Autodesk Inventor part; units mm, degrees
ref_plane "YZ Plane" through (0, 0, 0) normal (1, 0, 0) x (0, 1, 0)
ref_plane "XZ Plane" through (0, 0, 0) normal (0, 1, 0) x (-1, 0, 0)
ref_plane "XY Plane" through (0, 0, 0) normal (0, 0, 1) x (1, 0, 0)
sketch "Sketch1" plane through (0, 0, 0) normal (0, 1, 0) x (-1, 0, 0)
  line L0 (0, 0) -> (89, 0)
  line L1 (89, 0) -> (89, -94)
  line L2 (89, -94) -> (0, -94)
  line L3 (0, -94) -> (0, 0)
  dimension "d0" = 89
  dimension "d1" = 94
extrude "Extrusion1" add sketch "Sketch1" along normal blind 83
sketch "Sketch2" plane through (0, 83, 0) normal (0, 1, 0) x (1, 0, 0)
  line L0 (0, 0) -> (0, 2) construction
  line L1 (0, 0) -> (0, 94)
  line L2 (0, 2) -> (-2, 2) construction
  line L3 (-2, 2) -> (-87, 2)
  line L4 (-87, 2) -> (-87, 92)
  line L5 (-87, 92) -> (-2, 92)
  line L6 (-2, 92) -> (-2, 2)
  dimension "d4" = 2
  dimension "d5" = 2
  dimension "d6" = 85
  dimension "d7" = 90
extrude "Extrusion2" cut sketch "Sketch2" against normal blind 81
sketch "Sketch3" plane through (0, 2, 0) normal (0, 1, 0) x (1, 0, 0)
  line L0 (-87, 2) -> (-87, 92)
  line L1 (-87, 2) -> (-76, 2)
  line L2 (-2, 2) -> (-87, 2)
  line L3 (-76, 2) -> (-17, 2)
  line L4 (-87, 92) -> (-2, 92)
  line L5 (-76, 2) -> (-87, 2)
  line L6 (-87, 2) -> (-87, 92)
  line L7 (-87, 92) -> (-76, 92)
  line L8 (-2, 92) -> (-2, 2)
  line L9 (-17, 2) -> (-2, 2)
  line L10 (-2, 2) -> (-2, 92)
  line L11 (-2, 92) -> (-17, 92)
  line L12 (-87, 2) -> (-87, 17.5)
  line L13 (-87, 17.5) -> (-87, 76.5)
  line L14 (-87, 17.5) -> (-2, 17.5)
  line L15 (-2, 17.5) -> (-2, 2)
  line L16 (-2, 2) -> (-87, 2)
  line L17 (-87, 2) -> (-87, 17.5)
  line L18 (-87, 76.5) -> (-2, 76.5)
  line L19 (-2, 76.5) -> (-2, 92)
  line L20 (-2, 92) -> (-87, 92)
  line L21 (-87, 92) -> (-87, 76.5)
  point P0 (0, 0)
  point P1 (-2, 76.5)
  point P2 (-2, 17.5)
  dimension "d26" = 15.5
  dimension "d27" = 59
extrude "Extrusion3" add sketch "Sketch3" along normal blind 8 contours L0 L14 L8 L2 L1 | L0 L4 L8 L18
sketch "Sketch4" plane through (0, 2, 0) normal (0, 1, 0) x (1, 0, 0)
  line L0 (-46.5, 2) -> (43.5, 2) construction
  line L1 (-2, 17.5) -> (-87, 17.5)
  line L2 (-2, 17.5) -> (-6.5, 17.5)
  line L3 (-6.5, 17.5) -> (-6.5, 22.5)
  line L4 (-6.5, 22.5) -> (-2, 22.5)
  line L5 (-2, 22.5) -> (-2, 17.5)
  line L6 (-2, 76.5) -> (-2, 17.5)
  line L7 (-2, 76.5) -> (-6.5, 76.5)
  line L8 (-6.5, 76.5) -> (-6.5, 66.5)
  line L9 (-6.5, 66.5) -> (-2, 66.5)
  line L10 (-2, 66.5) -> (-2, 76.5)
  line L11 (-87, 17.5) -> (-81.2, 17.5)
  line L12 (-81.2, 17.5) -> (-81.2, 21.7)
  line L13 (-81.2, 21.7) -> (-87, 21.7)
  line L14 (-87, 21.7) -> (-87, 17.5)
  circle A0 centre (-81.2, 21.7) radius 1.35
  line L15 (-87, 17.5) -> (-87, 76.5)
  line L16 (-87, 47) -> (-2, 47) construction
  circle A1 centre (-81.2, 72.3) radius 1.35
  point P0 (-76, 2)
  dimension "d28" = 4.5
  dimension "d29" = 5
  dimension "d30" = 4.5
  dimension "d31" = 10
  dimension "d32" = 5.8
  dimension "d33" = 4.2
  dimension "d34" = 2.7
extrude "Extrusion4" add sketch "Sketch4" along normal blind 3 contours L9 L8 L7 L6 | L1 L3 L4 L5 | A0 L13 L12 | L12 L13 A0 | A1
sketch "Sketch6" plane through (-89, 0, -94) normal (-1, 0, 0) x (0, 0, 1)
  line L0 (0, 0) -> (0, 83)
  line L1 (0, 0) -> (2, 0) construction
  line L2 (2, 0) -> (2, 2) construction
  line L3 (2, 2) -> (0, 2) construction
  line L4 (0, 2) -> (0, 0)
  line L5 (2, 2) -> (27.5, 2) construction
  line L6 (20.35, 2) -> (20.35, 5)
  line L7 (2, 2) -> (27.5, 2) construction
  line L8 (27.5, 2) -> (27.5, 8.8) construction
  line L9 (27.5, 2) -> (34.3, 2) construction
  line L10 (27.5, 8.8) -> (41.5, 8.8)
  line L11 (41.5, 8.8) -> (41.5, 14.8)
  line L12 (41.5, 14.8) -> (27.5, 14.8)
  line L13 (27.5, 14.8) -> (27.5, 8.8)
  line L14 (94, 0) -> (92, 0) construction
  line L15 (92, 0) -> (92, 2) construction
  line L16 (92, 2) -> (94, 2) construction
  line L17 (94, 2) -> (94, 0) construction
  line L18 (92, 2) -> (76.5, 2) construction
  line L19 (76.5, 2) -> (71.5, 2) construction
  line L20 (71.5, 2) -> (71.5, 10) construction
  line L21 (71.5, 10) -> (60.5, 10)
  line L22 (60.5, 10) -> (60.5, 23)
  line L23 (60.5, 23) -> (71.5, 23)
  line L24 (71.5, 23) -> (71.5, 10)
  dimension "d35" = 2
  dimension "d36" = 2
  dimension "d37" = 25.5
  dimension "d38" = 0
  dimension "d39" = 6.8
  dimension "d40" = 90
  dimension "d41" = 14
  dimension "d42" = 6
  dimension "d43" = 2
  dimension "d44" = 2
  dimension "d45" = 15.5
  dimension "d46" = 5
  dimension "d47" = 8
  dimension "d48" = 11
  dimension "d49" = 13
extrude "Extrusion5" cut sketch "Sketch6" against normal up to surface (2 mm away)
sketch "Sketch7" plane through (0, 0, -94) normal (0, 0, -1) x (-1, 0, 0)
  line L0 (89, 83) -> (55.5, 83)
  line L1 (55.5, 83) -> (55.5, 34.3)
  line L2 (55.5, 34.3) -> (89, 34.3)
  line L3 (89, 34.3) -> (89, 83)
  line L4 (55.5, 34.3) -> (33.5, 34.3)
  line L5 (33.5, 34.3) -> (33.5, 30.2)
  line L6 (33.5, 30.2) -> (55.5, 30.2)
  line L7 (55.5, 30.2) -> (55.5, 34.3)
  line L8 (0, 0) -> (0, 83)
  point P0 (33.5, 32.25)
  dimension "d52" = 33.5
  dimension "d53" = 48.7
  dimension "d54" = 22
  dimension "d55" = 4.1
  dimension "d61" = 33.5
extrude "Extrusion6" cut sketch "Sketch7" against normal blind 1.1 contours L7 L6 L5 L4
sketch "Sketch8" plane through (-89, 0, 0) normal (0, 0, 1) x (1, 0, 0)
  line L0 (89, 0) -> (89, 83)
  line L1 (89, 83) -> (55.5, 83)
  line L2 (55.5, 83) -> (55.5, 34.3)
  line L3 (55.5, 34.3) -> (89, 34.3)
  line L4 (89, 34.3) -> (89, 83)
  line L5 (33.5, 30.2) -> (55.5, 30.2)
  line L6 (55.5, 34.3) -> (33.5, 34.3)
  line L7 (33.5, 34.3) -> (33.5, 30.2)
  line L8 (33.5, 30.2) -> (55.5, 30.2)
  line L9 (55.5, 30.2) -> (55.5, 34.3)
  dimension "d62" = 33.5
  dimension "d63" = 48.7
  dimension "d64" = 22
extrude "Extrusion7" cut sketch "Sketch8" against normal blind 1.1 contours L9 L5 L7 L6
properties part number "Arduino_case"
The model under review builds one solid part; all positions refer to its coordinate system, in mm. A direction names the side the tool comes from. Round coordinates to 2 decimals unless told otherwise and drop trailing zeros. Write each loop counter-clockwise with the first axis right and the second up, starting at its lowest first coordinate (ties: lowest second). Pieces come first, ordered by that corner, then holes. Notation, with made-up numbers: M 70,24 L 100,24 A30 ccw 100,51 Z; hole C 55.5,49.25 d7. An arc over 180 degrees is marked long. Use a Markdown table: item, result. Add a question column.
Q1. The part is to be moulded in two halves that separate along X. For faces 1 (the face through (0, 41, -48)), 2 (the face through (-45, 10, -10)), 3 (the face through (-44, 41, 0)), say which applies: pulls with the +X half, pulls with the -X half, needs draft (parallel to the pull), parting line crosses it, or undercut.
Q2. We need section B-B, the plane x = -81.2. State the section outline as (y, z) points, plus the area to 3 significant figures.
Q3. We need section C-C, the plane z = -11.5. State the section outline as (x, y) points, plus the area to 3 significant figures.
Q4. To check wall thickness, follow line 1 (X direction, y = 42, z = -4.5); line 2 (Z direction, x = -6.5, y = 66.5); line 3 (Z direction, x = -36.5, y = 8). State the ranges of each line that lie inside material, in increasing order.
Q5. Machinability: for faces 4 (the face through (-45, 32, -1.1)), 5 (the face through (-44, 47, -2)), which of the approach directions +Z, -Z, +X, -X, +Y, -Y give a long, thin tool a straight path to every point of the face, cutting with its end or side? Answer none if there is none.
Q6. We need section D-D, the plane y = 42.5. State the section outline as (x, z) points, plus the area to 3 significant figures.
Q7. We need section A-A, the plane z = -29.5. State the section outline as (x, y) points, plus the area to 3 significant figures.
Q8. Insertion check: pin 1 (1.5 mm diameter, centred on x = -15, z = -19.5, fed in from +Y); pin 2 (8 mm diameter, centred on x = -57.5, z = -82.5, fed in from +Y); pin 3 (1.3 mm diameter, centred on x = -4, z = -20, fed in from +Y). Each pin has a flat end and moves straight along its axis. Give the tip position at first contact, or say it passes through.
Findings below:
| question | item | result |
|---|---|---|
| 1 | face 1 | pulls with the +X half |
| 1 | face 2 | undercut |
| 1 | face 3 | needs draft |
| 2 | outline | M 0,-94 L 83,-94 L 83,-92 L 10,-92 L 10,-76.5 L 2,-76.5 L 2,-73.65 L 5,-73.65 L 5,-70.95 L 2,-70.95 L 2,-23.05 L 5,-23.05 L 5,-20.35 L 2,-20.35 L 2,-17.5 L 10,-17.5 L 10,-2 L 83,-2 L 83,0 L 0,0 Z |
| 2 | area | 776 mm² |
| 3 | outline | M -89,0 L 0,0 L 0,83 L -2,83 L -2,10 L -87,10 L -87,83 L -89,83 Z |
| 3 | area | 1,180 mm² |
| 4 | line 1 | x = -89 to -87, -2 to 0 |
| 4 | line 2 | z = -94 to -92, -2 to 0 |
| 4 | line 3 | z = -94 to -76.5, -17.5 to 0 |
| 5 | face 4 | +Z |
| 5 | face 5 | +Y |
| 6 | outline | M -89,-94 L 0,-94 L 0,0 L -89,0 Z; hole M -87,-92 L -2,-92 L -2,-2 L -87,-2 Z |
| 6 | area | 716 mm² |
| 7 | outline | M -89,0 L 0,0 L 0,83 L -2,83 L -2,2 L -87,2 L -87,10 L -89,10 Z; M -89,23 L -87,23 L -87,83 L -89,83 Z |
| 7 | area | 476 mm² |
| 8 | pin 1 | stops at y = 2 |
| 8 | pin 2 | stops at y = 10 |
| 8 | pin 3 | stops at y = 5 |
